Geometry: final body of the model. Coordinates: model frame, mm. Face numbers are marked on the shaded views. Give positions to 0.01 mm unless a question says otherwise; leave off trailing zeros. Write each loop counter-clockwise with the first axis right and the second up, starting at its lowest first coordinate (ties: lowest second). Pieces come first, ordered by that corner, then holes. Notation, with made-up numbers: (-18.5, -30.75) - (-7.5, -30.75) arc R21 ccw to (-7.5, -3.75) - close; hole circle Ø5 at (51.25, -36). An arc over 180 degrees is marked (long way). Return JSON: item names as keys, results as strings.
from build123d import *

# Parameters (mm, degrees)
F1_DEPTH = 870
F2_R     = 5
F3_R     = 5
F4_R     = 10
F5_DEPTH = 88.001


with BuildPart() as f1:
    # F0 (on Front) → F1 (new body)
    with BuildSketch(Plane.XZ):
        Polygon((-37.754953, -37.964115), (-12.754953, -37.964115), (-12.754953, -34.964115), (-34.754953, -34.964115), (-34.754953, 17.035885), (47.245047, 17.035885), (47.245047, -34.964115), (25.245047, -34.964115), (25.245047, -37.964115), (50.245047, -37.964115), (50.245047, 20.035885), (-37.754953, 20.035885), align=None)
    extrude(amount=F1_DEPTH)

    # F2
    f2_edges = [f1.edges().sort_by_distance(p)[0] for p in [
        (-37.754953, -435, 20.035885),
        (50.245047, -435, 20.035885),
        (-37.754953, -435, -37.964115),
        (50.245047, -435, -37.964115),
    ]]
    fillet(f2_edges, radius=F2_R)

    # F3
    f3_edges = [f1.edges().sort_by_distance(p)[0] for p in [
        (47.245047, -435, -34.964115),
        (47.245047, -435, 17.035885),
        (-34.754953, -435, -34.964115),
        (-34.754953, -435, 17.035885),
    ]]
    fillet(f3_edges, radius=F3_R)

    # F4 (on face) → F5 (cut, through all)
    with BuildSketch(Plane.YZ.offset(50.245047)):
        with Locations((-665, -8.964115)):
            Circle(F4_R)
        with Locations((-100, -8.964115)):
            Circle(F4_R)
    extrude(amount=-F5_DEPTH, mode=Mode.SUBTRACT)


solid = f1.part
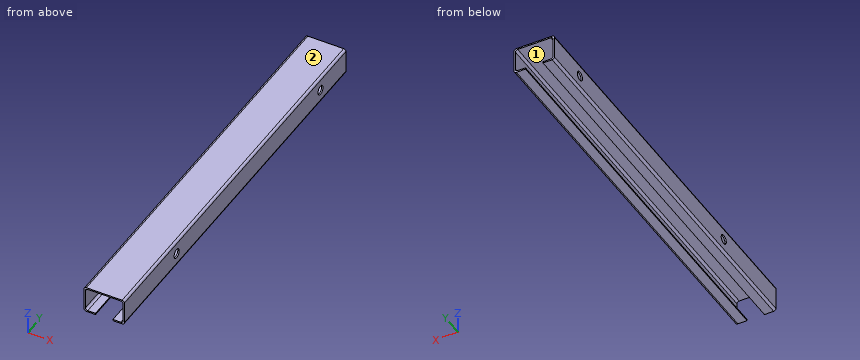
Q1. Material intervals for probe 1 along Z at (x, y) = (-19, -832.5); probe 2 along X at (y, z) = (-138, -23); probe 3 along X at (y, z) = (-746, 16), sorted ascending. Write a range as [from, to].
Answer key:
{"probe 1": "z = [-37.96, -34.96], [17.04, 20.04]", "probe 2": "x = [-37.75, -34.75], [47.25, 50.25]", "probe 3": "x = [-37.66, -32.8], [45.29, 50.15]"}
Q2. Mould query, pull axis X, two halves, no side actions, for the marked faces 1 and 2. Classes: pulls with the +X half, pulls with the -X half, needs draft (parallel to the pull), parting line crosses it, or undercut.
Answer key:
{"face 1": "undercut", "face 2": "needs draft"}
Q3. Section query A-A, the plane y = -100. Return the cut outline in (x, z), plus the area to 3 significant figures.
Answer key:
{"outline": "(-37.75, -32.96) arc R5 ccw to (-32.75, -37.96) - (-12.75, -37.96) - (-12.75, -34.96) - (-29.75, -34.96) arc R5 cw to (-34.75, -29.96) - (-34.75, -18.96) - (-37.75, -18.96) - close; (-37.75, 1.04) - (-34.75, 1.04) - (-34.75, 12.04) arc R5 cw to (-29.75, 17.04) - (42.25, 17.04) arc R5 cw to (47.25, 12.04) - (47.25, 1.04) - (50.25, 1.04) - (50.25, 15.04) arc R5 ccw to (45.25, 20.04) - (-32.75, 20.04) arc R5 ccw to (-37.75, 15.04) - close; (25.25, -37.96) - (45.25, -37.96) arc R5 ccw to (50.25, -32.96) - (50.25, -18.96) - (47.25, -18.96) - (47.25, -29.96) arc R5 cw to (42.25, -34.96) - (25.25, -34.96) - close", "area": "606 mm^2"}
Q4. Pin query (flat end, axial travel): P1, Ø2.5, axis at y = -550, z = -37, coming from the -X side; P2, Ø16, axis at y = -665, z = -8.96, coming from the -X side; P3, Ø6, axis at x = 7, y = -660.5, coming from the -Z side; P4, Ø2.5, axis at y = -399, z = -36.5, coming from the +X side. Return the tip coordinate at first contact, or that it passes through.
Answer key:
{"P1": "stops at x = -36.91", "P2": "passes through", "P3": "stops at z = 17.04", "P4": "stops at x = 49.69"}
Q5. Section query B-B, the plane x = 34.5. Return the cut outline in (y, z), plus the area to 3 significant figures.
Answer key:
{"outline": "(-870, -37.96) - (0, -37.96) - (0, -34.96) - (-870, -34.96) - close; (-870, 17.04) - (0, 17.04) - (0, 20.04) - (-870, 20.04) - close", "area": "5,220 mm^2"}
Q6. Section query C-C, the plane x = -4.5. Return the cut outline in (y, z), plus the area to 3 significant figures.
Answer key:
{"outline": "(-870, 17.04) - (0, 17.04) - (0, 20.04) - (-870, 20.04) - close", "area": "2,610 mm^2"}
